```python
from build123d import *

# Parameters (mm, degrees)
F0_W     = 240
F0_H     = 32
F1_DEPTH = 11.75
F4_DEPTH = 8
F5_W     = 21.1
F5_H     = 4
F6_DEPTH = 3.9
F7_W     = 130
F7_H     = 80
F8_DEPTH = 30
F9_R     = 5


with BuildPart() as f1:
    # F0 (on Front) → F1 (new body)
    with BuildSketch(Plane.XZ):
        Rectangle(F0_W, F0_H)
    extrude(amount=F1_DEPTH)

    # F3 (on face) → F4 (cut)
    with BuildSketch(Plane.XZ.offset(11.75)):
        Polygon((114.9, 10.58), (85.1, 10.58), (85.1, 3.325), (89.45, 3.325), (89.45, -10.75), (110.55, -10.75), (110.55, 3.325), (114.9, 3.325), align=None)
        Polygon((74.9, 10.58), (45.1, 10.58), (45.1, 3.325), (49.45, 3.325), (49.45, -10.75), (70.55, -10.75), (70.55, 3.325), (74.9, 3.325), align=None)
        Polygon((34.9, 10.58), (5.1, 10.58), (5.1, 3.325), (9.45, 3.325), (9.45, -10.75), (30.55, -10.75), (30.55, 3.325), (34.9, 3.325), align=None)
        Polygon((-5.1, 10.58), (-34.9, 10.58), (-34.9, 3.325), (-30.55, 3.325), (-30.55, -10.75), (-9.45, -10.75), (-9.45, 3.325), (-5.1, 3.325), align=None)
        Polygon((-45.1, 10.58), (-74.9, 10.58), (-74.9, 3.325), (-70.55, 3.325), (-70.55, -10.75), (-49.45, -10.75), (-49.45, 3.325), (-45.1, 3.325), align=None)
        Polygon((-85.1, 10.58), (-114.9, 10.58), (-114.9, 3.325), (-110.55, 3.325), (-110.55, -10.75), (-89.45, -10.75), (-89.45, 3.325), (-85.1, 3.325), align=None)
    extrude(amount=-F4_DEPTH, mode=Mode.SUBTRACT)

    # F5 (on face) → F6 (join)
    with BuildSketch(Plane.XZ.offset(3.75)):
        with Locations((100, -8.75)):
            Rectangle(F5_W, F5_H)
        with Locations((60, -8.75)):
            Rectangle(F5_W, F5_H)
        with Locations((20, -8.75)):
            Rectangle(F5_W, F5_H)
        with Locations((-20, -8.75)):
            Rectangle(F5_W, F5_H)
        with Locations((-60, -8.75)):
            Rectangle(F5_W, F5_H)
        with Locations((-100, -8.75)):
            Rectangle(F5_W, F5_H)
    extrude(amount=F6_DEPTH)

    # F7 (on Front) → F8 (cut)
    with BuildSketch(Plane.XZ):
        with Locations((-65, 0.10457)):
            Rectangle(F7_W, F7_H)
    extrude(amount=F8_DEPTH, mode=Mode.SUBTRACT)

    # F9
    f9_edges = [f1.edges().sort_by_distance(p)[0] for p in [
        (120, -5.875, -16),
        (120, -5.875, 16),
        (0, -5.875, -16),
        (0, -5.875, 16),
    ]]
    fillet(f9_edges, radius=F9_R)


solid = f1.part
```
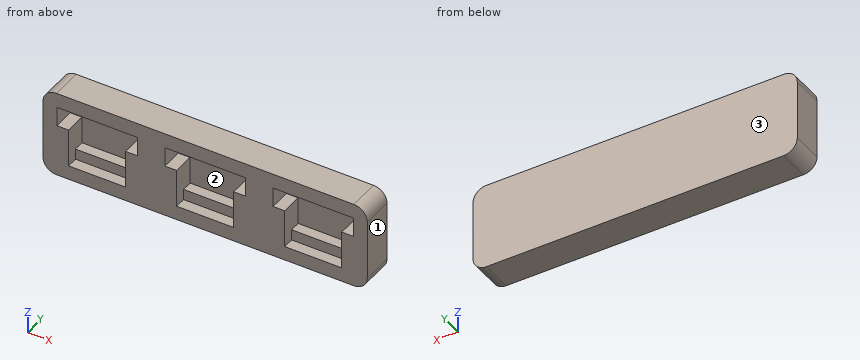
CAD build for the part. Positions are in the model's coordinates, mm. Face numbers are marked on the shaded views. Round coordinates to 2 decimals unless told otherwise and drop trailing zeros. Order: outer loops, then holes, each group sorted by start corner. A loop starts at its lowest first (then second) coordinate and runs counter-clockwise, first axis right, second up.
Q1. Wall check: L1, parallel to X at y = -9.5, z = 3; L2, parallel to X at y = -7.75, z = 8.5; L3, parallel to Z at x = 108, y = -4.75. Give the ranges that are in metal, low to high.
Q2. Slice it at B-B (x = 27.5). Write the cut outline in (y, z), and give its area (3 significant figures).
Q3. Slice it at C-C (z = 14). Write the cut outline in (x, y).
Q4. Two-plate mould, pull along X, no slides. Class the marked faces 1, 2 and 3: pulls with the +X half, pulls with the -X half, needs draft (parallel to the pull), parting line crosses it, or undercut.
Q5. Slice it at A-A (y = -6.25). State how many separate pieces and enclosed holes the cut face has, and give its area (3 significant figures).
Q6. Drop flat-ended pins along their axis: pin 1 (5 mm diameter, centred on x = 55, z = 2, fed in from -Y); pin 2 (3 mm diameter, centred on x = 57, z = -8, fed in from -Y). Give the stop position or say it passes through.
Results below:
1. L1: x = 0 to 9.45, 30.55 to 49.45, 70.55 to 89.45, 110.55 to 120
1. L2: x = 0 to 5.1, 34.9 to 45.1, 74.9 to 85.1, 114.9 to 120
1. L3: z = -16 to -6.75, 10.58 to 16
2. outline: (-11.75, -16) - (0, -16) - (0, 16) - (-11.75, 16) - (-11.75, 10.58) - (-3.75, 10.58) - (-3.75, -6.75) - (-7.65, -6.75) - (-7.65, -10.75) - (-11.75, -10.75) - close
2. area: 221 mm2
3. outline: (1, -11.75) - (119, -11.75) - (119, 0) - (1, 0) - close
4. face 1: pulls with the +X half
4. face 2: undercut
4. face 3: needs draft
5. separate pieces: 1
5. enclosed holes: 3
5. area: 2,530 mm2
6. pin 1: stops at y = -3.75
6. pin 2: stops at y = -7.65
